Design review of the part shown in the three views and the two pictorial views. Dimensions are in mm from the part's minimum x, y and z. A direction names the side the tool comes from. Give positions to 0.01 mm unless a question says otherwise; leave off trailing zeros. Write each loop counter-clockwise with the first axis right and the second up, starting at its lowest first coordinate (ties: lowest second). Pieces come first, ordered by that corner, then holes.
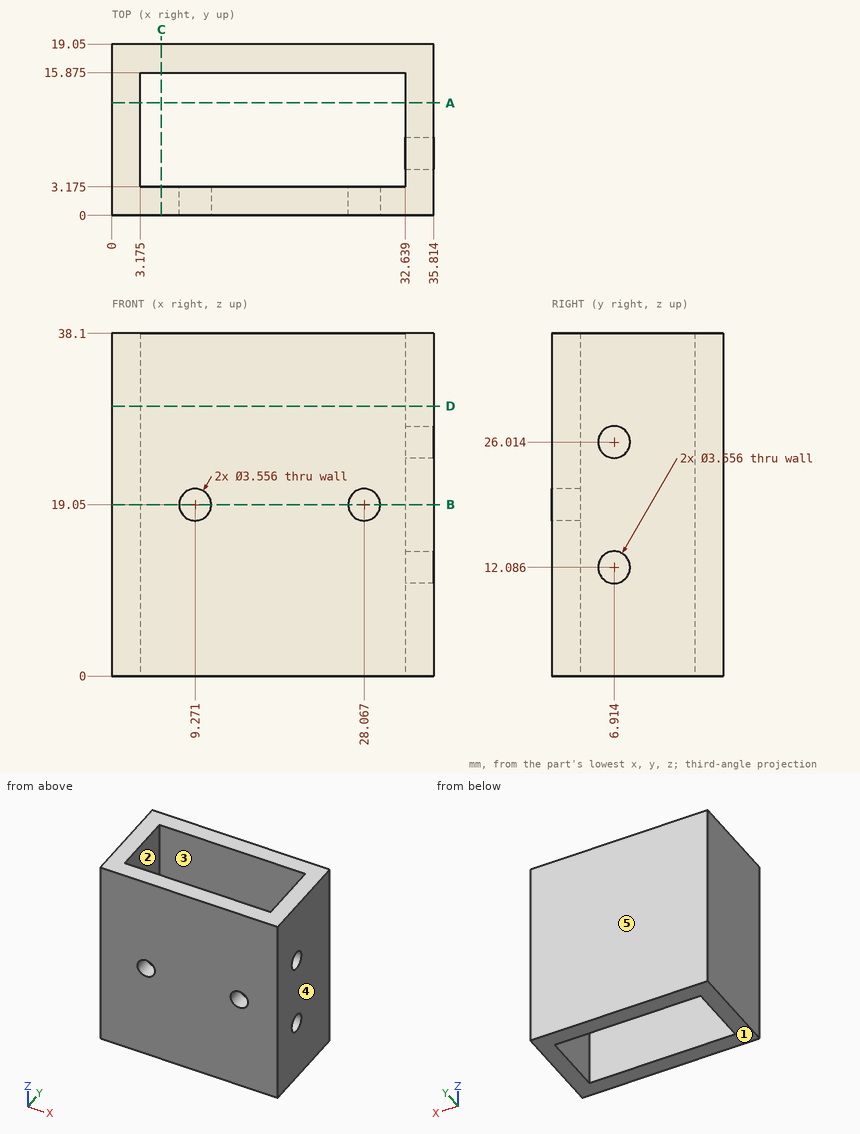
(1) Consider section A-A, the plane y = 12.5. Give the boundary of the cut face in (x, z) (3 decimals).
Resolved:
outline: (0, 0) - (3.175, 0) - (3.175, 38.1) - (0, 38.1) - close; (32.639, 0) - (35.814, 0) - (35.814, 38.1) - (32.639, 38.1) - close
(2) Consider section B-B, the plane z = 19.05. Give the boundary of the cut face in (x, y) (3 decimals).
Resolved:
outline: (0, 0) - (7.493, 0) - (7.493, 3.175) - (3.175, 3.175) - (3.175, 15.875) - (32.639, 15.875) - (32.639, 3.175) - (29.845, 3.175) - (29.845, 0) - (35.814, 0) - (35.814, 19.05) - (0, 19.05) - close; (11.049, 0) - (26.289, 0) - (26.289, 3.175) - (11.049, 3.175) - close
(3) Mouldability with a two-part tool opening along X and no side actions: class the marked faces 3, 4 and 5 as pulls with the +X half, pulls with the -X half, needs draft (parallel to the pull), parting line crosses it, or undercut.
Resolved:
face 3: undercut
face 4: pulls with the +X half
face 5: needs draft
(4) Clearance check with flat-ended pins moving along their axes: P1, Ø1.5, axis at x = 31, y = 10.5, coming from the -Z side; P2, Ø3, axis at y = 6.91, z = 12.09, coming from the +X side (3 decimals). State where each tip first meets the part, or that it passes through.
Resolved:
P1: passes through
P2: stops at x = 3.175
(5) To check wall thickness, follow L1, parallel to X at y = 1, z = 19.05 (3 decimals); L2, parallel to Y at x = 27.5, z = 5 (3 decimals); L3, parallel to X at y = 8, z = 7 (3 decimals). State the ranges of each line that lie inside material, in increasing order.
Resolved:
L1: x = 0 to 7.493, 11.049 to 26.289, 29.845 to 35.814
L2: y = 0 to 3.175, 15.875 to 19.05
L3: x = 0 to 3.175, 32.639 to 35.814
(6) Consider section D-D, the plane z = 30. Give the boundary of the cut face in (x, y) (3 decimals).
Resolved:
outline: (0, 0) - (35.814, 0) - (35.814, 19.05) - (0, 19.05) - close; hole (3.175, 3.175) - (32.639, 3.175) - (32.639, 15.875) - (3.175, 15.875) - close
(7) Consider section C-C, the plane x = 5.5. Give the boundary of the cut face in (y, z) (3 decimals).
Resolved:
outline: (0, 0) - (3.175, 0) - (3.175, 38.1) - (0, 38.1) - close; (15.875, 0) - (19.05, 0) - (19.05, 38.1) - (15.875, 38.1) - close
(8) Tool access review of the marked faces 1 and 2: name each direction out of +Z, -Z, +X, -X, +Y, -Y from which nothing blocks a thin tool from reaching the whole face with its end or side.
Resolved:
face 1: -Z, +X, -X, +Y, -Y
face 2: +Z, -Z
